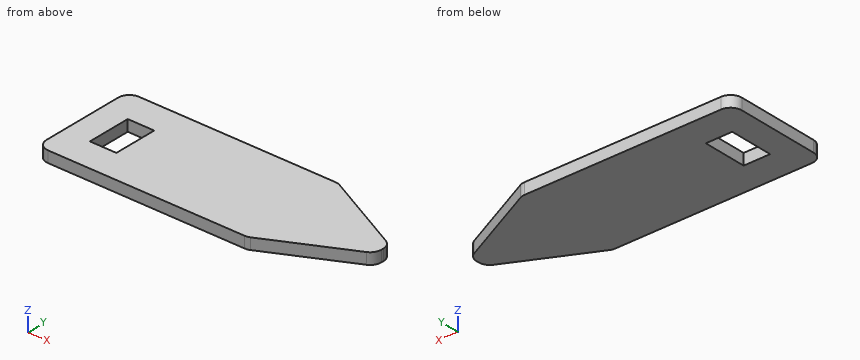
```python
from build123d import *

# Parameters (mm, degrees)
F0_W       = 3
F0_H       = 3.5
F0_W_2     = 25
F0_H_2     = 12
F1_DEPTH   = 1.27
F2_SIZE2   = 5.08
F2_SIZE    = 10.16
F2_2_SIZE2 = 5.08
F2_2_SIZE  = 10.16
F3_R       = 1.27
F4_R       = 1.27


with BuildPart() as f1:
    # F0 (on Top) → F1 (new body)
    with BuildSketch(Plane.XY):
        Polygon((-42.1337384582, -30.2597887341), (-45.1337384582, -30.2597887341), (-45.1337384582, -42.2597887341), (-42.1337384582, -42.2597887341), (-42.1337384582, -38.7597887341), (-42.1337384582, -33.7597887341), align=None)
        with Locations((-40.6337384582, -32.0097887341)):
            Rectangle(F0_W, F0_H)
        with Locations((-40.6337384582, -40.5097887341)):
            Rectangle(F0_W, F0_H)
        Polygon((-36.1337384582, -30.2597887341), (-39.1337384582, -30.2597887341), (-39.1337384582, -33.7597887341), (-39.1337384582, -38.7597887341), (-39.1337384582, -42.2597887341), (-36.1337384582, -42.2597887341), align=None)
        with Locations((-23.6337384582, -36.2597887341)):
            Rectangle(F0_W_2, F0_H_2)
    extrude(amount=F1_DEPTH)

    # F2
    f2_edges = [f1.edges().sort_by_distance(p)[0] for p in [
        (-11.133738, -30.259789, 0.635),
    ]]
    f2_side = f1.faces().sort_by_distance((-28.133738, -30.259789, 0.635))[0]
    chamfer(f2_edges, length=F2_SIZE, length2=F2_SIZE2, reference=f2_side)

    # F2#2
    f2_2_edges = [f1.edges().sort_by_distance(p)[0] for p in [
        (-11.133738, -42.259789, 0.635),
    ]]
    f2_2_side = f1.faces().sort_by_distance((-28.133738, -42.259789, 0.635))[0]
    chamfer(f2_2_edges, length=F2_2_SIZE, length2=F2_2_SIZE2, reference=f2_2_side)

    # F3
    f3_edges = [f1.edges().sort_by_distance(p)[0] for p in [
        (-21.293738, -30.259789, 0.635),
        (-11.133738, -35.339789, 0.635),
        (-11.133738, -37.179789, 0.635),
        (-21.293738, -42.259789, 0.635),
    ]]
    fillet(f3_edges, radius=F3_R)

    # F4
    f4_edges = [f1.edges().sort_by_distance(p)[0] for p in [
        (-45.133738, -42.259789, 0.635),
        (-45.133738, -30.259789, 0.635),
    ]]
    fillet(f4_edges, radius=F4_R)


solid = f1.part
```
Can you work these out from the model? Positions are in its coordinate system, mm. Coordinates: 2 decimals unless noted, no trailing zeros. Write each loop counter-clockwise with the first axis right and the second up, starting at its lowest first coordinate (ties: lowest second). Pieces come first, ordered by that corner, then holes. Notation, with made-up numbers: M 12.5,78 L 66.5,78 A21 ccw 66.5,91 Z; hole C 88.25,31 d1. An arc over 180 degrees is marked long. Write item = value, one per line. Start each with the question number.
Q1. If we section it at C-C, the plane y = -40.25: Write out the boundary of the cut face in (x, z).
Q2. If we section it at B-B, the plane y = -32.5: Write out the boundary of the cut face in (x, z).
Q3. If we section it at A-A, the plane z = 0.45: Write out the boundary of the cut face in (x, y).
Q4. If I drill on L1, parallel to Y at x = -39.5, z = 0.85; L2, parallel to X at y = -36, z = 0.1; L3, parallel to X at y = -37.5, z = 1, over which ranges is the centre line in solid material (lowest first)? Write a range as [from, to].
Q5. I'm going to push a flat-ended pin straight in: pin 1 (2 mm diameter, centred on x = -40.5, y = -40.5, fed in from -Z). Where does the tip first touch, or does it pass through?
Check sheet entries:
q1.outline = M -45.13,0 L -17.27,0 L -17.27,1.27 L -45.13,1.27 Z
q2.outline = M -45.13,0 L -16.81,0 L -16.81,1.27 L -45.13,1.27 Z
q3.outline = M -45.13,-40.99 A1.27 ccw -43.86,-42.26 L -21.59,-42.26 A1.27 ccw -21.03,-42.13 L -11.84,-37.53 A1.27 ccw -11.13,-36.39 L -11.13,-36.12 A1.27 ccw -11.84,-34.99 L -21.03,-30.39 A1.27 ccw -21.59,-30.26 L -43.86,-30.26 A1.27 ccw -45.13,-31.53 Z; hole M -42.13,-38.76 L -39.13,-38.76 L -39.13,-33.76 L -42.13,-33.76 Z
q4.L1 = [-42.26, -38.76], [-33.76, -30.26]
q4.L2 = [-45.13, -42.13], [-39.13, -11.14]
q4.L3 = [-45.13, -42.13], [-39.13, -11.78]
q5.pin_1 = 0
